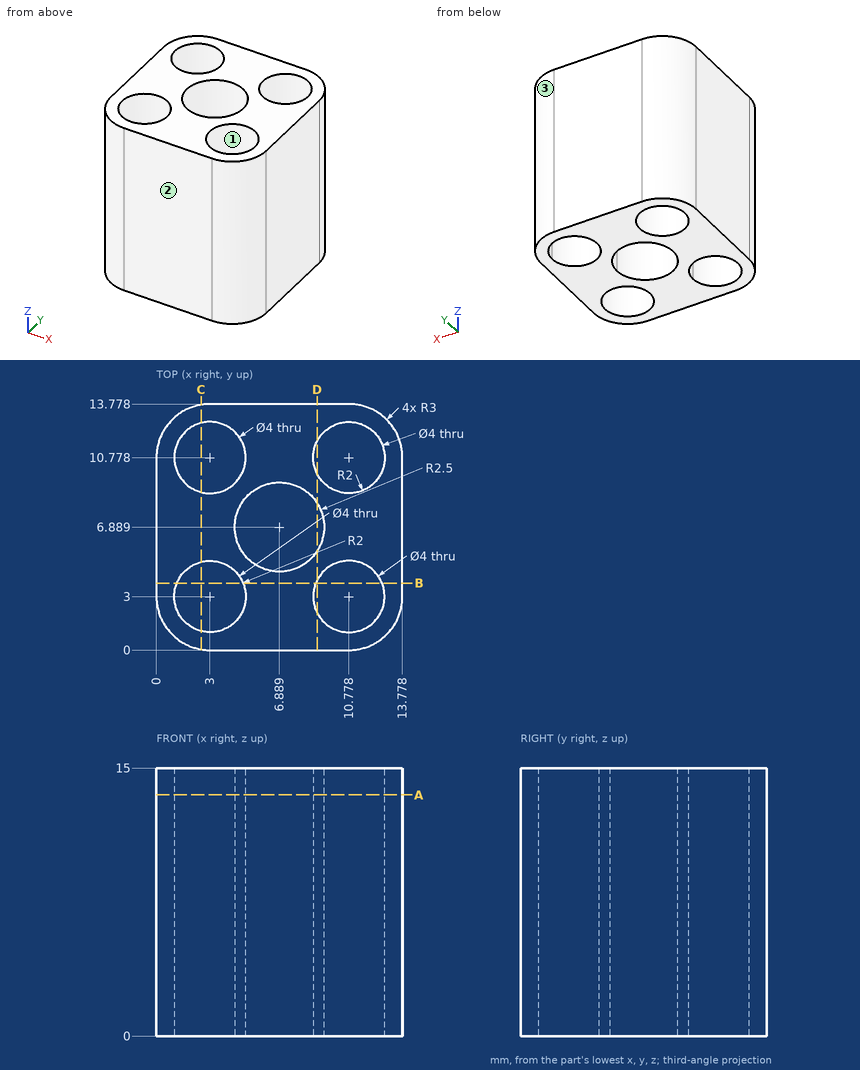
Source: three-view drawing plus pictorial views. Frame: mm from the lowest corner of the part. Give positions to 0.01 mm unless a question says otherwise; leave off trailing zeros. Loops run counter-clockwise (first coordinate to the right, second up) from the corner with the lowest first, then second, coordinate; pieces in that order, holes last.
1) Line query: L1, parallel to X at y = 10.75, z = 11; L2, parallel to X at y = 2.5, z = 12 (1 decimal); L3, parallel to X at y = 7.25, z = 6.5 (1 decimal). Output: solid intervals per line, ascending.
A:
L1: x = 0 to 1, 5 to 8.78, 12.78 to 13.78
L2: x = 0 to 1.1, 4.9 to 8.8, 12.7 to 13.7
L3: x = 0 to 4.4, 9.4 to 13.8
2) Section query A-A on z = 13.5. Return the cut outline in (x, y), and give its area (3 significant figures).
A:
outline: (0, 3) arc R3 ccw to (3, 0) - (10.78, 0) arc R3 ccw to (13.78, 3) - (13.78, 10.78) arc R3 ccw to (10.78, 13.78) - (3, 13.78) arc R3 ccw to (0, 10.78) - close; hole circle Ø4 at (3, 10.78); hole (4.41, 4.41) arc R2 ccw (long way) to (5, 3) arc R2 ccw to start; hole (8.66, 8.66) arc R2.5 ccw (long way) to (9.39, 6.89) arc R2.5 ccw to start; hole circle Ø4 at (10.78, 3); hole circle Ø4 at (10.78, 10.78)
area: 112 mm2
3) Section query D-D on x = 9. Return the cut outline in (y, z).
A:
outline: (0, 0) - (2.08, 0) - (2.08, 15) - (0, 15) - close; (3.92, 0) - (5.55, 0) - (5.55, 15) - (3.92, 15) - close; (8.23, 0) - (9.86, 0) - (9.86, 15) - (8.23, 15) - close; (11.69, 0) - (13.78, 0) - (13.78, 15) - (11.69, 15) - close
4) Section query C-C on x = 2.5. Return the cut outline in (y, z) (1 decimal).
A:
outline: (0, 0) - (1.1, 0) - (1.1, 15) - (0, 15) - close; (4.9, 0) - (8.8, 0) - (8.8, 15) - (4.9, 15) - close; (12.7, 0) - (13.7, 0) - (13.7, 15) - (12.7, 15) - close
5) Contact query for a flat-ended pin moving along its axis: pin 1 (3 mm diameter, centred on x = 12.5, z = 2, fed in from -Y). Output: stop coordinate, or through.
A:
pin 1: stops at y = 0.01
6) Section query B-B on y = 3.75. Return the cut outline in (x, z).
A:
outline: (0, 0) - (1.15, 0) - (1.15, 15) - (0, 15) - close; (4.85, 0) - (8.92, 0) - (8.92, 15) - (4.85, 15) - close; (12.63, 0) - (13.78, 0) - (13.78, 15) - (12.63, 15) - close
7) Mould query, pull axis X, two halves, no side actions, for the marked faces 1, 2 and 3. Classes: released by +X, released by -X, zero draft, split by the parting line, or undercut.
A:
face 1: undercut
face 2: zero draft
face 3: released by +X
